The drawing under review shows one solid part. Ordinate dimensions are in mm from its lowest x, y, z. Coordinates: 2 decimals unless noted, no trailing zeros. Loops run counter-clockwise (first coordinate to the right, second up) from the corner with the lowest first, then second, coordinate; pieces in that order, holes last. Notation, with made-up numbers: M 56.5,-10.75 L 113.5,-10.75 A30 cw 113.5,16.25 Z; hole C -25.75,60 d6. An arc over 180 degrees is marked long. Return JSON: item names as keys, results as strings.
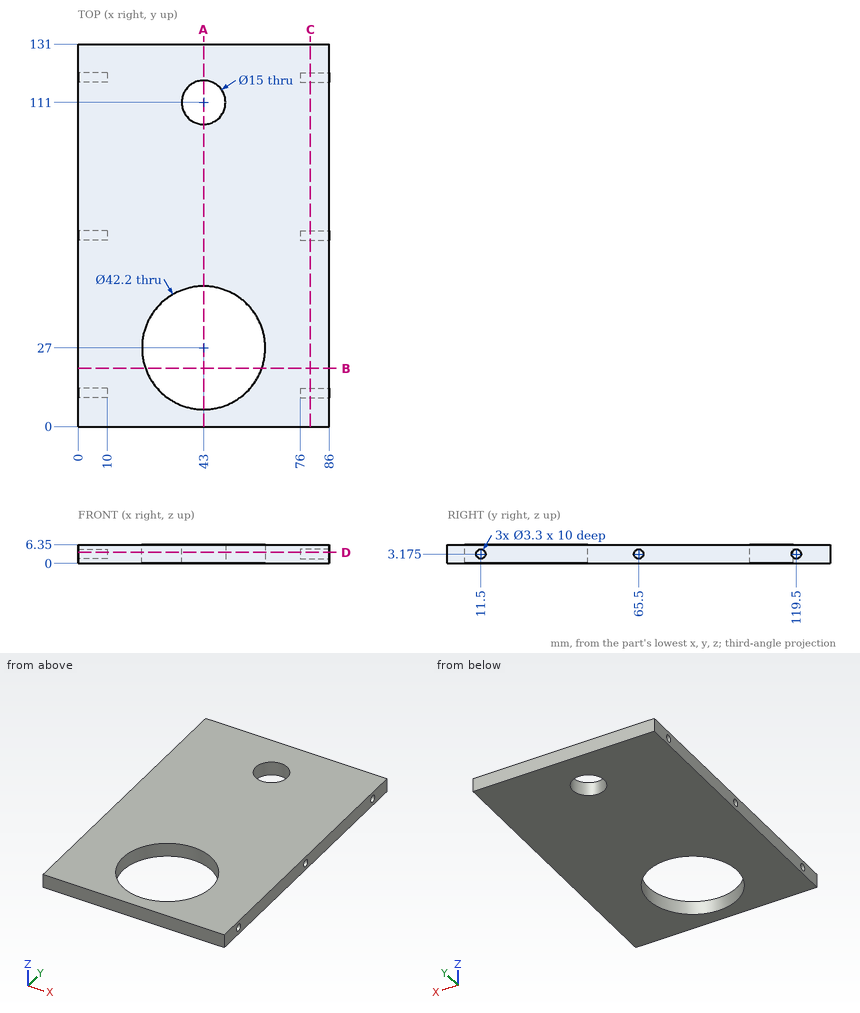
1. Add section C-C on x = 79.5. Give the boundary of the cut face in (y, z) (3 decimals).
Check values:
{"outline": "M 0,0 L 131,0 L 131,6.35 L 0,6.35 Z; hole C 11.5,3.175 d3.3; hole C 65.5,3.175 d3.3; hole C 119.5,3.175 d3.3"}
2. To check wall thickness, follow line 1 (Z direction, x = 84.25, y = 11.5) (3 decimals); line 2 (Y direction, x = 9, z = 2); line 3 (Y direction, x = 40, z = 2.5). State the ranges of each line that lie inside material, in increasing order.
Check values:
{"line 1": "0 to 1.525, 4.825 to 6.35", "line 2": "0 to 10.34, 12.66 to 64.34, 66.66 to 118.34, 120.66 to 131", "line 3": "0 to 6.11, 47.89 to 104.13, 117.87 to 131"}
3. Add section A-A on x = 43. Give the boundary of the cut face in (y, z).
Check values:
{"outline": "M 0,0 L 5.9,0 L 5.9,6.35 L 0,6.35 Z; M 48.1,0 L 103.5,0 L 103.5,6.35 L 48.1,6.35 Z; M 118.5,0 L 131,0 L 131,6.35 L 118.5,6.35 Z"}
4. Add section B-B on y = 20. Give the boundary of the cut face in (x, z).
Check values:
{"outline": "M 0,0 L 23.09,0 L 23.09,6.35 L 0,6.35 Z; M 62.91,0 L 86,0 L 86,6.35 L 62.91,6.35 Z"}
5. Add section D-D on z = 3.75. State how many separate pieces and enclosed holes the cut face has, plus the area to 3 significant figures.
Check values:
{"separate pieces": "1", "enclosed holes": "2", "area": "9,510 mm²"}
6. Insertion check: pin 1 Ø1 at (y, z) = (65, 3.5) entering from +X; pin 2 Ø1.6 at (y, z) = (120, 3) entering from -X. Each pin has a flat end and moves straight along its axis. Give the tip position at first contact, or say it passes through.
Check values:
{"pin 1": "x = 76", "pin 2": "x = 10"}
